Source: three-view drawing plus pictorial views. Frame: mm from the lowest corner of the part. Give positions to 0.01 mm unless a question says otherwise; leave off trailing zeros. Loops run counter-clockwise (first coordinate to the right, second up) from the corner with the lowest first, then second, coordinate; pieces in that order, holes last. Notation, with made-up numbers: M -32.75,24.5 L -13.75,24.5 A15 ccw -13.75,53.5 Z; hole C -0.75,26.5 d3. An arc over 180 degrees is marked long. One line per item, written item: value. Start each with the question number.
(1) Ray query, line 1 along Y through (x, z) = (13, 2.2) (1 decimal). Return the intervals inside material, ascending. Write a range as from..to.
(2) Section B-B on y = 44. Output: boundary loops of the cut face in (x, z) (1 decimal).
(3) Section A-A on z = 0.7. Output: boundary loops of the cut face in (x, y) (1 decimal).
(4) Pin query (flat end, axial travel): P1, Ø1.4, axis at x = 62.5, z = 1.5, coming from the -Y side; P2, Ø5, axis at x = 59.5, y = 13, coming from the -Z side; P3, Ø0.9, axis at x = 11, z = 1, coming from the +Y side; P4, Ø1.4, axis at y = 2, z = 1, coming from the -X side. Return the tip coordinate at first contact, or that it passes through.
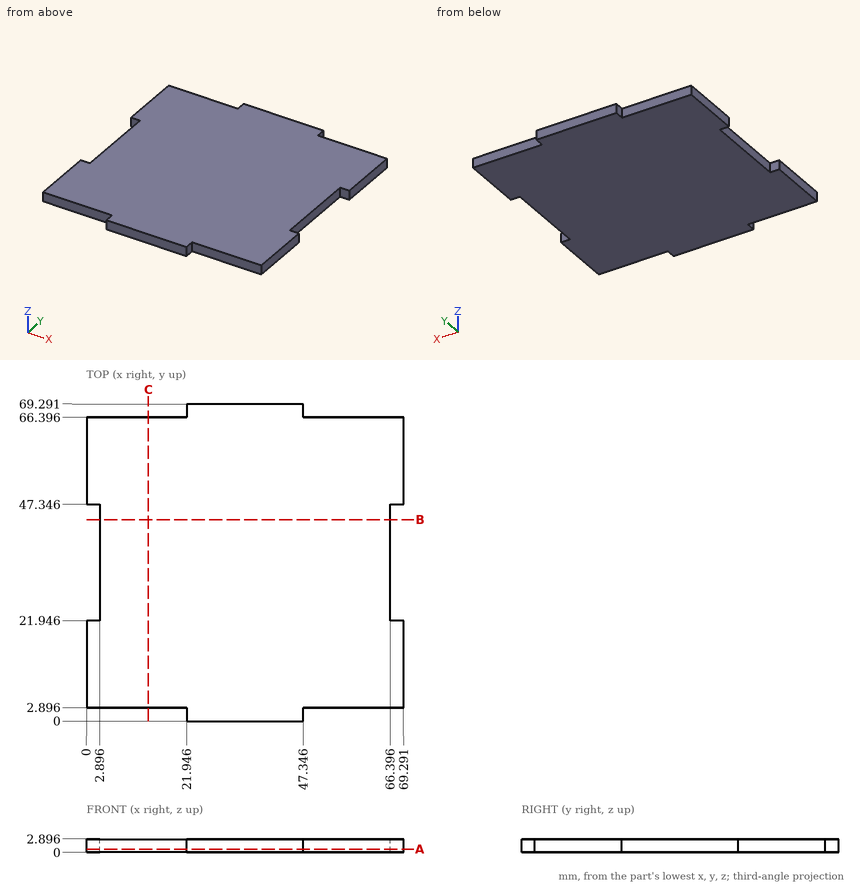
Output values:
1. line 1: y = 2.9..66.4
2. outline: M 2.9,0 L 66.4,0 L 66.4,2.9 L 2.9,2.9 Z
3. outline: M 0,2.9 L 21.9,2.9 L 21.9,0 L 47.3,0 L 47.3,2.9 L 69.3,2.9 L 69.3,21.9 L 66.4,21.9 L 66.4,47.3 L 69.3,47.3 L 69.3,66.4 L 47.3,66.4 L 47.3,69.3 L 21.9,69.3 L 21.9,66.4 L 0,66.4 L 0,47.3 L 2.9,47.3 L 2.9,21.9 L 0,21.9 Z
4. P1: stops at y = 2.9
4. P2: stops at z = 0
4. P3: stops at y = 66.4
4. P4: stops at x = 21.95
